Check sheet for the modelled part. Datum: model origin and axes. Units: mm. A direction names the side the tool comes from. Give positions to 0.01 mm unless a question says otherwise; leave off trailing zeros. Order: outer loops, then holes, each group sorted by start corner. A loop starts at its lowest first (then second) coordinate and runs counter-clockwise, first axis right, second up. Notation, with made-up numbers: (-9, 31) -> (35, 31) arc R19 ccw to (35, 50) -> close; hole circle Ø8 at (27, 35.25). An arc over 180 degrees is marked (long way). Answer in a Markdown table with one row per item. Add a question column.
(1) Set-up check for faces 4 (the face through (45.03, 5.59, -37.36)), 5 (the face through (47.8, 5, -35)), 6 (the face through (-1, 0, -1)): record each of +Z, -Z, +X, -X, +Y, -Y from which the full face is reachable in a straight line by a thin tool's end or side.
(2) Cross-section at C-C (z = -35). Record the cut outline in (x, y).
(3) Go/stop test with flat-tipped pins: pin 1 (3 mm diameter, centred on y = 7, z = -33.5, fed in from -X); pin 2 (12 mm diameter, centred on x = 22.5, z = -7.5, fed in from +Y); pin 3 (1.2 mm diameter, centred on x = -46.5, y = 5.5, fed in from +Z). Record where each tip stops, or that it passes through.
(4) Cross-section at A-A (z = 0). Record the cut outline in (x, y), then the cut area to 3 significant figures.
(5) Thickness scan on L1, parallel to Y at x = 47.45, z = 35; L2, parallel to Y at x = 20.5, z = 16; L3, parallel to X at y = 36.5, z = -6.5. Record the ranges inside material, lowest first. Write a range as [from, to].
(6) Release check for a two-part mould opening along Z. For faces 1 (the face through (46, 7, 30)), 2 (the face through (-43.8, 4.7, -32.7)), 3 (the face through (-9.76, 41.44, -2.17)) record: released by +Z, released by -Z, zero draft, split by the parting line, or undercut.
(7) Cross-section at D-D (y = 59.5). Record the cut outline in (x, z).
(8) Cross-section at B-B (x = 0). Record the cut outline in (y, z).
```python
from build123d import *

# Parameters (mm, degrees)
IZIM1_W                     = 100
IZIM1_H                     = 100
Y_KSEKLIK_EKSTR_ZYON1_DEPTH = 2
IZIM2_R                     = 10
Y_KSEKLIK_EKSTR_ZYON2_DEPTH = 80
IZIM3_W                     = 4
IZIM3_H                     = 10
Y_KSEKLIK_EKSTR_ZYON3_DEPTH = 10
KES_EKSTR_ZYON1_DEPTH       = 2.5
IZIM6_R                     = 1.6
KES_EKSTR_ZYON2_DEPTH       = 5
KES_EKSTR_ZYON3_DEPTH       = 2.5
KES_EKSTR_ZYON4_START       = -5
IZIM8_R                     = 1.6
KES_EKSTR_ZYON4_DEPTH       = 5


with BuildPart() as part:
    # Çizim1 → Yükseklik-Ekstrüzyon1 (new body)
    with BuildSketch(Plane(origin=(0, 0, 0), x_dir=(1, 0, 0), z_dir=(0, 1, 0))):
        Rectangle(IZIM1_W, IZIM1_H)
    extrude(amount=Y_KSEKLIK_EKSTR_ZYON1_DEPTH)

    # Çizim2 → Yükseklik-Ekstrüzyon2 (add)
    with BuildSketch(Plane(origin=(0, 2, 0), x_dir=(1, 0, 0), z_dir=(0, 1, 0))):
        with Locations(Location((0, 0, 0), (0, 0, 270))):
            Circle(IZIM2_R)
    extrude(amount=Y_KSEKLIK_EKSTR_ZYON2_DEPTH)

    # Çizim3 → Yükseklik-Ekstrüzyon3 (add)
    with BuildSketch(Plane(origin=(0, 2, 0), x_dir=(1, 0, 0), z_dir=(0, 1, 0))):
        with Locations((-45.8, 35)):
            Rectangle(IZIM3_W, IZIM3_H)
        with Locations((45.8, 35)):
            Rectangle(IZIM3_W, IZIM3_H)
        with Locations((-45.8, -35)):
            Rectangle(IZIM3_W, IZIM3_H)
        with Locations((45.8, -35)):
            Rectangle(IZIM3_W, IZIM3_H)
    extrude(amount=Y_KSEKLIK_EKSTR_ZYON3_DEPTH)

    # Çizim5 → Kes-Ekstrüzyon1 (cut)
    with BuildSketch(Plane(origin=(-43.8, 0, 0), x_dir=(0, 0, -1), z_dir=(1, 0, 0))):
        Polygon((-36.526149852, 4.215363585), (-33.35150905, 4.285997251), (-31.825359198, 7.070633666), (-33.473850148, 9.784636415), (-36.64849095, 9.714002749), (-38.174640802, 6.929366334), align=None)
        Polygon((33.473850148, 4.215363585), (36.64849095, 4.285997251), (38.174640802, 7.070633666), (36.526149852, 9.784636415), (33.35150905, 9.714002749), (31.825359198, 6.929366334), align=None)
    extrude(amount=-KES_EKSTR_ZYON1_DEPTH, mode=Mode.SUBTRACT)

    # Çizim6 → Kes-Ekstrüzyon2 (cut)
    with BuildSketch(Plane(origin=(-43.8, 0, 0), x_dir=(0, 0, -1), z_dir=(1, 0, 0))):
        with Locations((-35, 7)):
            Circle(IZIM6_R)
        with Locations((35, 7)):
            Circle(IZIM6_R)
    extrude(amount=-KES_EKSTR_ZYON2_DEPTH, mode=Mode.SUBTRACT)

    # Çizim7 → Kes-Ekstrüzyon3 (cut)
    with BuildSketch(Plane.ZY.offset(-43.8)):
        Polygon((-33.475734775, 9.785668476), (-36.650327054, 9.712886645), (-38.174592279, 6.927218169), (-36.524265225, 4.214331524), (-33.349672946, 4.287113355), (-31.825407721, 7.072781831), align=None)
        Polygon((36.524265225, 9.785668476), (33.349672946, 9.712886645), (31.825407721, 6.927218169), (33.475734775, 4.214331524), (36.650327054, 4.287113355), (38.174592279, 7.072781831), align=None)
    extrude(amount=-KES_EKSTR_ZYON3_DEPTH, mode=Mode.SUBTRACT)

    # Çizim8 → Kes-Ekstrüzyon4 (cut)
    with BuildSketch(Plane.ZY.offset(-43.8).offset(KES_EKSTR_ZYON4_START)):
        with Locations(Location((35, 7, 0), (0, 0, 180))):
            Circle(IZIM8_R)
        with Locations(Location((-35, 7, 0), (0, 0, 180))):
            Circle(IZIM8_R)
    extrude(amount=KES_EKSTR_ZYON4_DEPTH, mode=Mode.SUBTRACT)


solid = part.part
```
Answer below:
| question | item | result |
|---|---|---|
| 1 | face 4 | none |
| 1 | face 5 | +Z, -Z, +X, +Y |
| 1 | face 6 | +Z, -Z, +X, -X, -Y |
| 2 | outline | (-50, 0) -> (50, 0) -> (50, 2) -> (47.8, 2) -> (47.8, 5.4) -> (46.3, 5.4) -> (46.3, 4.25) -> (43.8, 4.25) -> (43.8, 2) -> (-43.8, 2) -> (-43.8, 4.25) -> (-46.3, 4.25) -> (-46.3, 5.4) -> (-47.8, 5.4) -> (-47.8, 2) -> (-50, 2) -> close; (-47.8, 8.6) -> (-46.3, 8.6) -> (-46.3, 9.75) -> (-43.8, 9.75) -> (-43.8, 12) -> (-47.8, 12) -> close; (43.8, 9.75) -> (46.3, 9.75) -> (46.3, 8.6) -> (47.8, 8.6) -> (47.8, 12) -> (43.8, 12) -> close |
| 3 | pin 1 | stops at x = -47.8 |
| 3 | pin 2 | stops at y = 2 |
| 3 | pin 3 | stops at z = 40 |
| 4 | outline | (-50, 0) -> (50, 0) -> (50, 2) -> (10, 2) -> (10, 82) -> (-10, 82) -> (-10, 2) -> (-50, 2) -> close |
| 4 | area | 1,800 mm² |
| 5 | L1 | y = [0, 5.4], [8.6, 12] |
| 5 | L2 | y = [0, 2] |
| 5 | L3 | x = [-7.6, 7.6] |
| 6 | face 1 | undercut |
| 6 | face 2 | zero draft |
| 6 | face 3 | split by the parting line |
| 7 | outline | circle Ø20 at (0, 0) |
| 8 | outline | (0, -50) -> (2, -50) -> (2, -10) -> (82, -10) -> (82, 10) -> (2, 10) -> (2, 50) -> (0, 50) -> close |
